Work out the finished part from the listing and answer in its coordinate system (mm). Face numbers are marked on the shaded views. A direction names the side the tool comes from. Coordinates: 2 decimals unless noted, no trailing zeros. Write each loop counter-clockwise with the first axis right and the second up, starting at its lowest first coordinate (ties: lowest second). Pieces come first, ordered by that corner, then holes. Notation, with made-up numbers: (67, -35) - (125, -35) arc R14 ccw to (125, -13) - close; hole circle Ø8 at (8.25, 57). An arc over 180 degrees is marked (long way). Use a Markdown table: item, result. Add a question column.
(1) A tool of negligible diameter and unlimited length cuts with its end or side. For the marked faces 1 and 2, from which of +Z, -Z, +X, -X, +Y, -Y can it reach the whole face along a straight path? Write none if from no direction.
(2) The part is cut by section A-A, the plane x = 4.5. Give the vertices of the cut face in (y, z), then the cut area to 4 significant figures.
(3) Find the intervals of material crossed by line 1 (Z direction, x = 7.5, y = 83); line 2 (Z direction, x = -1, y = 129); line 3 (X direction, y = 47, z = 1.5), in increasing order. Write a range as from..to.
(4) Given pin 1 Ø5 at (x, z) = (7, -29) entering from -Y; pin 2 Ø1 at (y, z) = (47.5, -27.5) entering from +X; pin 3 Ø0.9 at (x, y) = (1, 80) entering from -Z, each flat-ended and moving along its own axis, determine where each tip first touches the part or whether it passes through.
(5) The part is cut by section C-C, the plane z = -5. Give the vertices of the cut face in (x, y).
(6) The part is cut by section B-B, the plane y = 55. Give the vertices of the cut face in (x, z), then the cut area to 3 significant figures.
(7) For a pull along Y with two mould halves and no side action, classify the marked faces 3 and 4 as released by +Y, released by -Y, zero draft, split by the parting line, or undercut.
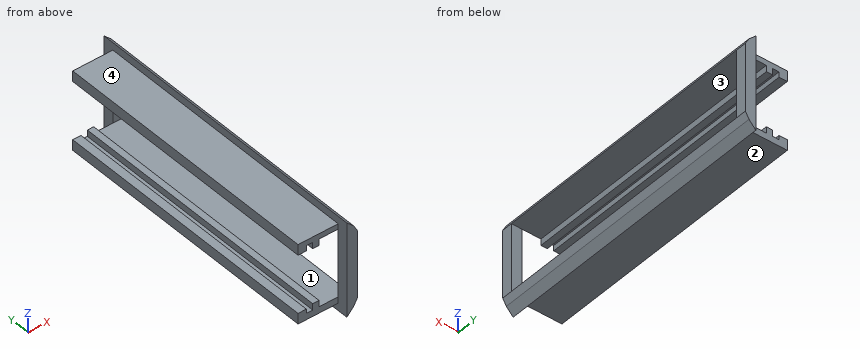
from build123d import *

# Parameters (mm, degrees)
BOSS_EXTRUDE2_DEPTH = 130
BOSS_EXTRUDE3_DEPTH = 5
BOSS_EXTRUDE4_DEPTH = 5
CUT_EXTRUDE2_DEPTH  = 6


with BuildPart() as part:
    # Sketch1 → Boss-Extrude2 (new body)
    with BuildSketch(Plane(origin=(0, 0, 0), x_dir=(1, 0, 0), z_dir=(0, 1, 0))):
        Polygon((0, -3), (0, 29), (3, 29), (3, 26), (6, 26), (6, 29), (20, 29), (18.290622359, 32), (15.075355057, 35.5), (15.075355057, 32), (-3.924644943, 32), (-3.924644943, -5.5), (15.075355057, -5.5), (15.075355057, -9), (18.290622359, -6), (20, -3), (6, -3), (6, 0), (3, 0), (3, -3), align=None)
    extrude(amount=BOSS_EXTRUDE2_DEPTH)

    # Sketch2 → Boss-Extrude3 (add)
    with BuildSketch(Plane(origin=(0, 130, 0), x_dir=(1, 0, 0), z_dir=(0, 1, 0))):
        Polygon((15.075355057, 35.5), (15.075355057, -9), (18.290622359, -6), (20, -3), (20, 29), (18.290622359, 32), align=None)
    extrude(amount=BOSS_EXTRUDE3_DEPTH)

    # Sketch3 → Boss-Extrude4 (add)
    with BuildSketch(Plane.XZ):
        Polygon((15.075355057, 9), (15.075355057, -35.5), (18.290622359, -32), (20, -29), (20, 3), (18.290622359, 6), align=None)
    extrude(amount=BOSS_EXTRUDE4_DEPTH)

    # Sketch4 → Cut-Extrude2 (cut)
    with BuildSketch(Plane.ZY.offset(3.924644943)):
        Polygon((0.5, 5), (0.5, 125), (0.5, 130), (-27, 130), (-27, 125), (-27, 5), (-27, 0), (0.5, 0), align=None)
    extrude(amount=-CUT_EXTRUDE2_DEPTH, mode=Mode.SUBTRACT)


solid = part.part
Model answer:
| question | item | result |
|---|---|---|
| 1 | face 1 | +X |
| 1 | face 2 | -Z, -X, +Y, -Y |
| 2 | outline | (0, -32) - (130, -32) - (130, -26) - (0, -26) - close; (0, 0) - (130, 0) - (130, 5.5) - (0, 5.5) - close |
| 2 | area | 1,495 mm^2 |
| 3 | line 1 | -32..-29, 3..5.5 |
| 3 | line 2 | -32..-27, 0.5..5.5 |
| 3 | line 3 | -3.92..0, 3..6 |
| 4 | pin 1 | y = 0 |
| 4 | pin 2 | x = 6 |
| 4 | pin 3 | z = -32 |
| 5 | outline | (15.08, -5) - (20, -5) - (20, 0) - (15.08, 0) - close; (15.08, 130) - (20, 130) - (20, 135) - (15.08, 135) - close |
| 6 | outline | (-3.92, -32) - (15.08, -32) - (15.08, -35.5) - (18.29, -32) - (20, -29) - (6, -29) - (6, -26) - (3, -26) - (3, -29) - (0, -29) - (0, -27) - (-3.92, -27) - close; (-3.92, 0.5) - (0, 0.5) - (0, 3) - (3, 3) - (3, 0) - (6, 0) - (6, 3) - (20, 3) - (18.29, 6) - (15.08, 9) - (15.08, 5.5) - (-3.92, 5.5) - close |
| 6 | area | 175 mm^2 |
| 7 | face 3 | undercut |
| 7 | face 4 | zero draft |
